```python
from build123d import *

# Parameters (mm, degrees)
SKETCH_W      = 16
SKETCH_H      = 6
SKETCH_W_2    = 6.05
SKETCH_H_2    = 3.05
PAD_DEPTH     = 2.05
SKETCH001_W   = 16
SKETCH001_H   = 6
PAD001_DEPTH  = 1.45
SKETCH002_W   = 16
SKETCH002_H   = 160
SKETCH002_W_2 = 6.05
SKETCH002_H_2 = 3.05
PAD002_DEPTH  = 4
SKETCH003_R   = 1.7
HOLE_DEPTH    = 25
SKETCH004_R   = 2
POCKET_DEPTH  = 1


with BuildPart() as part:
    # Sketch → Pad (new body)
    with BuildSketch(Plane.XY):
        Rectangle(SKETCH_W, SKETCH_H)
        with Locations((3.675, -0.475)):
            Rectangle(SKETCH_W_2, SKETCH_H_2, mode=Mode.SUBTRACT)
        with Locations((-3.675, -0.475)):
            Rectangle(SKETCH_W_2, SKETCH_H_2, mode=Mode.SUBTRACT)
    extrude(amount=PAD_DEPTH)

    # Sketch001 (on Face14 of Pad) → Pad001 (join)
    with BuildSketch(Plane.XY.offset(2.05)):
        Rectangle(SKETCH001_W, SKETCH001_H)
    extrude(amount=PAD001_DEPTH)

    # Sketch002 (on Face1 of Pad001) → Pad002 (join)
    with BuildSketch(Plane(origin=(0, 0, 0), x_dir=(1, 0, 0), z_dir=(0, 0, -1))):
        with Locations((0, -77)):
            Rectangle(SKETCH002_W, SKETCH002_H)
        with Locations((-3.675, 0.475)):
            Rectangle(SKETCH002_W_2, SKETCH002_H_2, mode=Mode.SUBTRACT)
        with Locations((3.675, 0.475)):
            Rectangle(SKETCH002_W_2, SKETCH002_H_2, mode=Mode.SUBTRACT)
    extrude(amount=PAD002_DEPTH)

    # Sketch003 (on Face3 of Pad002) → Hole (cut)
    with BuildSketch(Plane.XY):
        with Locations((4, 97)):
            Circle(SKETCH003_R)
        with Locations((-4, 97)):
            Circle(SKETCH003_R)
        with Locations((4, 17)):
            Circle(SKETCH003_R)
        with Locations((-4, 17)):
            Circle(SKETCH003_R)
        with Locations((4, 57)):
            Circle(SKETCH003_R)
        with Locations((-4, 57)):
            Circle(SKETCH003_R)
        with Locations((-4, 137)):
            Circle(SKETCH003_R)
        with Locations((4, 137)):
            Circle(SKETCH003_R)
    extrude(amount=-HOLE_DEPTH, mode=Mode.SUBTRACT)

    # Sketch004 (on Face3 of Hole) → Pocket (cut)
    with BuildSketch(Plane.XZ.offset(3)):
        with Locations((-3.675, -0.975)):
            Circle(SKETCH004_R)
        with Locations((3.675, -0.975)):
            Circle(SKETCH004_R)
    extrude(amount=-POCKET_DEPTH, mode=Mode.SUBTRACT)


solid = part.part
```
For this review, take the finished solid that the model builds, in its own axes (mm). A direction names the side the tool comes from. Coordinates: 2 decimals unless noted, no trailing zeros. Order: outer loops, then holes, each group sorted by start corner. A loop starts at its lowest first (then second) coordinate and runs counter-clockwise, first axis right, second up. Notation, with made-up numbers: (-21, -9) - (-14, -9) arc R15 ccw to (-14, 8) - close; hole circle Ø7 at (85.25, -11.75). An arc over 180 degrees is marked (long way). Answer as a JSON object with one key per item and string values. Group by question number.
1. We need section A-A on y = 137. State the section outline as (x, z) points, then the cut area to 3 significant figures.
2. We need section B-B on x = 4.25. Give the number of separate pieces and of enclosed holes in the cut face, then the cut area to 3 significant figures.
3. Clearance check with flat-ended pins moving along their axes: P1, Ø5, axis at x = 3.5, y = 125, coming from the +Z side; P2, Ø1.5, axis at x = 4.5, y = -0.5, coming from the -Z side; P3, Ø3, axis at x = -0.5, z = 2, coming from the +Y side. State where each tip first meets the part, or that it passes through.
4. For faces 4 (the cylindrical face through (4.914, 58.433, -1.972)), 5 (the flat face through (-4, 1.05, -1)), 6 (the flat face through (0, 79, 0)), list the 3-axis set-ups (+Z, -Z, +X, -X, +Y, -Y) from which the entire face can be reached by the end or side of a thin tool; tool diameter is ignored.
5. We need section C-C on y = 13. State the section outline as (x, z) points, then the cut area to 3 significant figures.
6. For probe 1 along X at (y, z) = (137, -0.9); probe 2 along Y at (x, z) = (4, -2.9); probe 3 along Y at (x, z) = (-1.5, -1.25), list the stretches that pass through material, from the lowest coordinate up.
7. The part is to be moulded in two halves that separate along Z. For faces 1 (the cylindrical face through (-2.43, 16.35, -1.97)), 2 (the flat face through (0, 0, 3.5)), 3 (the cylindrical face through (5.58, -2.51, -0.37)), say which applies: pulls with the +Z half, pulls with the -Z half, needs draft (parallel to the pull), parting line crosses it, or undercut.
Final values:
{
 "1": {"outline": "(-8, -4) - (-5.7, -4) - (-5.7, 0) - (-8, 0) - close; (-2.3, -4) - (2.3, -4) - (2.3, 0) - (-2.3, 0) - close; (5.7, -4) - (8, -4) - (8, 0) - (5.7, 0) - close", "area": "36.8 mm²"},
 "2": {"separate pieces": "6", "enclosed holes": "0", "area": "585 mm²"},
 "3": {"P1": "z = 0", "P2": "z = 2.05", "P3": "y = 3"},
 "4": {"face 4": "+Z, -Z", "face 5": "-Z", "face 6": "+Z, +X, -X, +Y"},
 "5": {"outline": "(-8, -4) - (8, -4) - (8, 0) - (-8, 0) - close", "area": "64.0 mm²"},
 "6": {"probe 1": "-8 to -5.7, -2.3 to 2.3, 5.7 to 8", "probe 2": "1.05 to 15.3, 18.7 to 55.3, 58.7 to 95.3, 98.7 to 135.3, 138.7 to 157", "probe 3": "-3 to -2, 1.05 to 157"},
 "7": {"face 1": "needs draft", "face 2": "pulls with the +Z half", "face 3": "undercut"}
}
